```python
from build123d import *

# Parameters (mm, degrees)
CROQUIS1_R              = 4
SALIENTE_EXTRUIR1_DEPTH = 5
CROQUIS2_R              = 5.5
CROQUIS2_R_2            = 3.5
SALIENTE_EXTRUIR2_DEPTH = 6
CROQUIS3_R              = 2.5
SALIENTE_EXTRUIR3_DEPTH = 11
CROQUIS4_R              = 2
SALIENTE_EXTRUIR4_DEPTH = 16
CROQUIS5_R              = 0.75
CORTAR_EXTRUIR1_DEPTH   = 6.5


with BuildPart() as part:
    # Croquis1 → Saliente-Extruir1 (new body)
    with BuildSketch(Plane.XY):
        Circle(CROQUIS1_R)
    extrude(amount=SALIENTE_EXTRUIR1_DEPTH)

    # Croquis2 → Saliente-Extruir2 (add)
    with BuildSketch(Plane.XY.offset(5)):
        Circle(CROQUIS2_R)
        Circle(CROQUIS2_R_2, mode=Mode.SUBTRACT)
    extrude(amount=SALIENTE_EXTRUIR2_DEPTH)

    # Croquis3 → Saliente-Extruir3 (add)
    with BuildSketch(Plane(origin=(0, 0, 0), x_dir=(-1, 0, 0), z_dir=(0, 0, -1))):
        Circle(CROQUIS3_R)
    extrude(amount=SALIENTE_EXTRUIR3_DEPTH)

    # Croquis4 → Saliente-Extruir4 (add)
    with BuildSketch(Plane(origin=(0, 0, -11), x_dir=(-1, 0, 0), z_dir=(0, 0, -1))):
        Circle(CROQUIS4_R)
    extrude(amount=SALIENTE_EXTRUIR4_DEPTH)

    # Croquis5 → Cortar-Extruir1 (cut, through all)
    with BuildSketch(Plane(origin=(0, 0, 0), x_dir=(1, 0, 0), z_dir=(0, 1, 0))):
        with Locations((0, 9.5)):
            Circle(CROQUIS5_R)
    extrude(amount=-CORTAR_EXTRUIR1_DEPTH, mode=Mode.SUBTRACT)


solid = part.part
```
The listing builds one solid part. Answer for the finished solid, in the listing's coordinates (mm). A direction names the side the tool comes from. Coordinates: 2 decimals unless noted, no trailing zeros. Write each loop counter-clockwise with the first axis right and the second up, starting at its lowest first coordinate (ties: lowest second). Pieces come first, ordered by that corner, then holes.
Q1. Section C-C, the plane y = 0.5 is taken. Write down the section's boundary in (x, z).
Returned:
outline: (-5.48, 5) - (-3.97, 5) - (-3.97, 0) - (-2.45, 0) - (-2.45, -11) - (-1.94, -11) - (-1.94, -27) - (1.94, -27) - (1.94, -11) - (2.45, -11) - (2.45, 0) - (3.97, 0) - (3.97, 5) - (5.48, 5) - (5.48, 11) - (3.46, 11) - (3.46, 5) - (-3.46, 5) - (-3.46, 11) - (-5.48, 11) - close
Q2. Section B-B, the plane z = -13 is taken. Write down the section's boundary in (x, y), then the cut area to 3 significant figures.
Returned:
outline: circle Ø4 at (0, 0)
area: 12.6 mm2
Q3. The mould has two halves that part along X. Classify faces 4 (the cylindrical face through (-1.34, 2.11, -5.42)), 5 (the flat face through (4, 0, 11)), 6 (the cylindrical face through (-0.098, -1.234, -10.244)): released by +X, released by -X, zero draft, split by the parting line, or undercut.
Returned:
face 4: split by the parting line
face 5: zero draft
face 6: undercut
Q4. Given P1, Ø0.8, axis at x = 0, z = -9.5, coming from the -Y side; P2, Ø6, axis at x = -4.5, z = -3.5, coming from the +Y side; P3, Ø6, axis at y = 0.5, z = -2.5, coming from the -X side, each flat-ended and moving along its own axis, determine where each tip first touches the part or whether it passes through.
Returned:
P1: stops at y = 0
P2: stops at y = 2
P3: stops at x = -4
Q5. Find the intervals of material crossed by line 1 along Y through (x, z) = (0, 9.6); line 2 along Z through (x, y) = (0, -1.5); line 3 along Z through (x, y) = (3.5, -3.25), in increasing order.
Returned:
line 1: y = -5.5 to -3.5, 3.5 to 5.5
line 2: z = -27 to -10.25, -8.75 to 5
line 3: z = 5 to 11
Q6. Section A-A, the plane x = 0 is taken. Write down the section's boundary in (y, z), then the cut area to 3 significant figures.
Returned:
outline: (-5.5, 5) - (-4, 5) - (-4, 0) - (-2.5, 0) - (-2.5, -8.75) - (0, -8.75) - (0, -10.25) - (-2.5, -10.25) - (-2.5, -11) - (-2, -11) - (-2, -27) - (2, -27) - (2, -11) - (2.5, -11) - (2.5, 0) - (4, 0) - (4, 5) - (5.5, 5) - (5.5, 11) - (3.5, 11) - (3.5, 5) - (-3.5, 5) - (-3.5, 11) - (-5.5, 11) - close
area: 179 mm2
Q7. Section D-D, the plane z = 7 is taken. Write down the section's boundary in (x, y), then the cut area to 3 significant figures.
Returned:
outline: circle Ø11 at (0, 0); hole circle Ø7 at (0, 0)
area: 56.5 mm2
Q8. Which of the six approach directions +Z, -Z, +X, -X, +Y, -Y give full straight-line access (tool end or side, diameter ignored) to faces 1 (the flat face through (0, 0, -10)), 2 (the flat face through (2, 2, 0)), 3 (the cylindrical face through (3.233, -1.341, 7.958))?
Returned:
face 1: -Y
face 2: -Z
face 3: +Z
